from build123d import *

# Parameters (mm, degrees)
SKETCH1_W           = 120
SKETCH1_H           = 80
SKETCH1_R           = 2.5
SKETCH1_R_2         = 11
BOSS_EXTRUDE1_DEPTH = 6.35
FILLET1_R           = 2


with BuildPart() as part:
    # Sketch1 → Boss-Extrude1 (new body)
    with BuildSketch(Plane.XY):
        Rectangle(SKETCH1_W, SKETCH1_H)
        with Locations((-50, 30)):
            Circle(SKETCH1_R, mode=Mode.SUBTRACT)
        with Locations((-30, 30)):
            Circle(SKETCH1_R, mode=Mode.SUBTRACT)
        with Locations((-10, 30)):
            Circle(SKETCH1_R, mode=Mode.SUBTRACT)
        with Locations((10, 30)):
            Circle(SKETCH1_R, mode=Mode.SUBTRACT)
        with Locations((30, 30)):
            Circle(SKETCH1_R, mode=Mode.SUBTRACT)
        with Locations((50, 30)):
            Circle(SKETCH1_R, mode=Mode.SUBTRACT)
        with Locations((-50, 10)):
            Circle(SKETCH1_R, mode=Mode.SUBTRACT)
        with Locations((50, 10)):
            Circle(SKETCH1_R, mode=Mode.SUBTRACT)
        with Locations((0, -10)):
            Circle(SKETCH1_R_2, mode=Mode.SUBTRACT)
    extrude(amount=BOSS_EXTRUDE1_DEPTH)

    # Fillet1
    fillet1_edges = [part.edges().sort_by_distance(p)[0] for p in [
        (60, -40, 3.175),
        (-60, -40, 3.175),
        (-60, 40, 3.175),
        (60, 40, 3.175),
    ]]
    fillet(fillet1_edges, radius=FILLET1_R)


solid = part.part
Geometry check sheet. Reference: the model listing, model coordinates, mm. Round coordinates to 2 decimals unless told otherwise and drop trailing zeros. Loops run counter-clockwise (first coordinate to the right, second up) from the corner with the lowest first, then second, coordinate; pieces in that order, holes last. Notation, with made-up numbers: (-35, 76.5) -> (-8, 76.5) arc R19 cw to (-8, 86.5) -> close; hole circle Ø11 at (-13, 0.25). An arc over 180 degrees is marked (long way). Answer as a JSON object with one key per item and string values. Group by question number.
Item 1: Thickness scan on line 1 along Y through (x, z) = (50, 6.25); line 2 along Y through (x, z) = (30, 2.75); line 3 along Y through (x, z) = (10, 2.25). Record the ranges inside material, lowest first.
Item 2: Cross-section at B-B, the plane y = -10. Record the cut outline in (x, z).
Item 3: Cross-section at D-D, the plane y = 10. Record the cut outline in (x, z).
Item 4: Cross-section at A-A, the plane x = 30. Record the cut outline in (y, z).
Item 5: Cross-section at C-C, the plane x = 50. Record the cut outline in (y, z), plus the area to 4 significant figures.
Item 6: Depth check by flat-ended pin: pin 1 Ø3 at (x, y) = (50, 10) entering from +Z. Enter the tip coordinate at first touch or a pass-through.
Item 7: Release check for a two-part mould opening along Y. For faces 1 (the face through (60, -1, 3)), 2 (the face through (28.16, 31.69, 3.13)), 3 (the face through (-1, 40, 3)) record: pulls with the +Y half, pulls with the -Y half, needs draft (parallel to the pull), parting line crosses it, or undercut.
Determined:
{
 "1": {"line 1": "y = -40 to 7.5, 12.5 to 27.5, 32.5 to 40", "line 2": "y = -40 to 27.5, 32.5 to 40", "line 3": "y = -40 to -14.58, -5.42 to 27.5, 32.5 to 40"},
 "2": {"outline": "(-60, 0) -> (-11, 0) -> (-11, 6.35) -> (-60, 6.35) -> close; (11, 0) -> (60, 0) -> (60, 6.35) -> (11, 6.35) -> close"},
 "3": {"outline": "(-60, 0) -> (-52.5, 0) -> (-52.5, 6.35) -> (-60, 6.35) -> close; (-47.5, 0) -> (47.5, 0) -> (47.5, 6.35) -> (-47.5, 6.35) -> close; (52.5, 0) -> (60, 0) -> (60, 6.35) -> (52.5, 6.35) -> close"},
 "4": {"outline": "(-40, 0) -> (27.5, 0) -> (27.5, 6.35) -> (-40, 6.35) -> close; (32.5, 0) -> (40, 0) -> (40, 6.35) -> (32.5, 6.35) -> close"},
 "5": {"outline": "(-40, 0) -> (7.5, 0) -> (7.5, 6.35) -> (-40, 6.35) -> close; (12.5, 0) -> (27.5, 0) -> (27.5, 6.35) -> (12.5, 6.35) -> close; (32.5, 0) -> (40, 0) -> (40, 6.35) -> (32.5, 6.35) -> close", "area": "444.5 mm²"},
 "6": {"pin 1": "passes through"},
 "7": {"face 1": "needs draft", "face 2": "undercut", "face 3": "pulls with the +Y half"}
}
